from build123d import *

# Parameters (mm, degrees)
SALIENTE_EXTRUIR2_DEPTH = 3


with BuildPart() as part:
    # Croquis1 → Saliente-Extruir2 (new body)
    with BuildSketch(Plane(origin=(0, 0, 0), x_dir=(1, 0, 0), z_dir=(0, 1, 0))):
        Polygon((3, 12.5), (3, 27.5), (0, 27.5), (0, 40), (17.5, 40), (17.5, 37), (32.5, 37), (32.5, 40), (47.5, 40), (47.5, 37), (62.5, 37), (62.5, 40), (77.5, 40), (77.5, 37), (92.5, 37), (92.5, 40), (110, 40), (110, 27.5), (107, 27.5), (107, 12.5), (110, 12.5), (110, 0), (92.5, 0), (92.5, 3), (77.5, 3), (77.5, 0), (62.5, 0), (62.5, 3), (47.5, 3), (47.5, 0), (32.5, 0), (32.5, 3), (17.5, 3), (17.5, 0), (0, 0), (0, 12.5), align=None)
    extrude(amount=SALIENTE_EXTRUIR2_DEPTH)


solid = part.part
Could you check a few things on this model? Use its own coordinates, in mm. A direction names the side the tool comes from. Coordinates: 2 decimals unless noted, no trailing zeros. Write each loop counter-clockwise with the first axis right and the second up, starting at its lowest first coordinate (ties: lowest second). Pieces come first, ordered by that corner, then holes. Notation, with made-up numbers: (49.5, 80.25) - (104.5, 80.25) arc R23 cw to (104.5, 100.25) - close; hole circle Ø2 at (-8.5, 68.5). An arc over 180 degrees is marked (long way). Write item = value, one per line.
1) For faces 1 (the flat face through (108, 1, -12.5)), 2 (the flat face through (32.5, 1, -38)), 3 (the flat face through (62.5, 1, -1)), which set-ups out of +Z, -Z, +X, -X, +Y, -Y let a thin tool reach every point of the face, with its end or its side?
Result set:
face_1 = +X, +Y, -Y
face_2 = -Z, +Y, -Y
face_3 = +Z, +Y, -Y
2) We'd pull the mould along X, two halves only. Please class faces 4 (the flat face through (109, 1, -27.5)), 5 (the flat face through (92.5, 1, -1)), 6 (the flat face through (107, 1, -20)), 7 (the flat face through (32.5, 1, -1)): +X half, -X half, draft (parallel to the pull), parting line (faces both ways), or undercut.
Result set:
face_4 = draft
face_5 = undercut
face_6 = +X half
face_7 = undercut
3) Suppose I cut it at B-B on x = 52.5. Please give me the cut outline in (y, z), plus the area to 3 significant figures.
Result set:
outline = (0, -37) - (3, -37) - (3, -3) - (0, -3) - close
area = 102 mm2
4) Please list where these lines run through material, in increasing order: line 1 (X direction, y = 2.55, z = -1.5); line 2 (X direction, y = 1.45, z = -25); line 3 (Z direction, x = 51, y = 2.45). Write a range as [from, to].
Result set:
line_1 = [0, 17.5], [32.5, 47.5], [62.5, 77.5], [92.5, 110]
line_2 = [3, 107]
line_3 = [-37, -3]
5) Will these pins go through, and if not, where does the flat tip stop? pin 1 Ø1 at (y, z) = (2, -21.5) entering from -X; pin 2 Ø1 at (y, z) = (2, -26) entering from +X; pin 3 Ø1.5 at (x, y) = (28.5, 1) entering from +Z.
Result set:
pin_1 = 3
pin_2 = 107
pin_3 = -3
6) Suppose I cut it at A-A on z = -26. Please give me the cut outline in (x, y), plus the area to 3 significant figures.
Result set:
outline = (3, 0) - (107, 0) - (107, 3) - (3, 3) - close
area = 312 mm2
